Model file for the job. Use its own axes, mm. Coordinates: 2 decimals unless noted, no trailing zeros. Write each loop counter-clockwise with the first axis right and the second up, starting at its lowest first coordinate (ties: lowest second). Pieces come first, ordered by that corner, then holes.
Q1. Pull direction Y, two halves, no side cores. Call faces 1 (the flat face through (99, 0, 2)), 2 (the flat face through (99, 41, 2)), 3 (the flat face through (99, 41, 0)), 4 (the flat face through (99, 80, 2)): released by +Y, released by -Y, zero draft, split by the parting line, or undercut.
Q2. Drill centre lines: probe 1 along X at (y, z) = (64, 1.7); probe 2 along Y at (x, z) = (36, 3.35); probe 3 along Z at (x, y) = (10, 45). Where is each one in solid material? Low to high.
Q3. Band-saw the part on A-A, the plane y = 10. Write the cut outline in (x, z), plus the area to 3 significant figures.
Q4. Band-saw the part on B-B, the plane z = 2.65. Write the cut outline in (x, y).
Q5. Band-saw the part on C-C, the plane x = 116. State how many separate pieces and enclosed holes the cut face has, plus the area to 3 significant figures.
from build123d import *

# Parameters (mm, degrees)
SKETCH_W      = 200
SKETCH_H      = 80
PAD_DEPTH     = 2
SKETCH001_W   = 158
SKETCH001_H   = 2
SKETCH001_W_2 = 156.797272
PAD001_DEPTH  = 2
SKETCH002_W   = 166
SKETCH002_H   = 8
SKETCH002_H_2 = 10
SKETCH002_H_3 = 12
SKETCH002_W_2 = 20
SKETCH002_H_4 = 4
SKETCH002_W_3 = 16
SKETCH002_W_4 = 22
SKETCH002_W_5 = 14
SKETCH002_W_6 = 18
SKETCH002_W_7 = 12
SKETCH002_H_5 = 6
POCKET_DEPTH  = 5


with BuildPart() as part:
    # Sketch → Pad (new body)
    with BuildSketch(Plane.XY):
        with Locations((100, 40)):
            Rectangle(SKETCH_W, SKETCH_H)
    extrude(amount=PAD_DEPTH)

    # Sketch001 (on Face6 of Pad) → Pad001 (join)
    with BuildSketch(Plane.XY.offset(2)):
        with Locations((101, 1)):
            Rectangle(SKETCH001_W, SKETCH001_H)
        with Locations((100.398636, 79)):
            Rectangle(SKETCH001_W_2, SKETCH001_H)
    extrude(amount=PAD001_DEPTH)

    # Sketch002 (on Face5 of Pad001) → Pocket (cut)
    with BuildSketch(Plane.XY.offset(2)):
        with Locations((99, 72)):
            Rectangle(SKETCH002_W, SKETCH002_H)
        with Locations((99, 61)):
            Rectangle(SKETCH002_W, SKETCH002_H_2)
        with Locations((99, 48)):
            Rectangle(SKETCH002_W, SKETCH002_H_3)
        with Locations((99, 8)):
            Rectangle(SKETCH002_W, SKETCH002_H)
        with Locations((26, 16)):
            Rectangle(SKETCH002_W_2, SKETCH002_H_4)
        with Locations((48, 16)):
            Rectangle(SKETCH002_W_3, SKETCH002_H_4)
        with Locations((73, 16)):
            Rectangle(SKETCH002_W_4, SKETCH002_H_4)
        with Locations((95, 16)):
            Rectangle(SKETCH002_W_5, SKETCH002_H_4)
        with Locations((115, 16)):
            Rectangle(SKETCH002_W_6, SKETCH002_H_4)
        with Locations((137, 16)):
            Rectangle(SKETCH002_W_6, SKETCH002_H_4)
        with Locations((156, 16)):
            Rectangle(SKETCH002_W_7, SKETCH002_H_4)
        with Locations((174, 16)):
            Rectangle(SKETCH002_W_3, SKETCH002_H_4)
        with Locations((99, 25)):
            Rectangle(SKETCH002_W, SKETCH002_H_5)
        with Locations((99, 35)):
            Rectangle(SKETCH002_W, SKETCH002_H_5)
    extrude(amount=-POCKET_DEPTH, mode=Mode.SUBTRACT)


solid = part.part
Answer sheet:
1. face 1: released by -Y
1. face 2: undercut
1. face 3: zero draft
1. face 4: released by +Y
2. probe 1: x = 0 to 16, 182 to 200
2. probe 2: y = 0 to 2, 78 to 80
2. probe 3: z = 0 to 2
3. outline: (0, 0) - (16, 0) - (16, 2) - (0, 2) - close; (182, 0) - (200, 0) - (200, 2) - (182, 2) - close
3. area: 68.0 mm2
4. outline: (22, 0) - (180, 0) - (180, 2) - (22, 2) - close; (22, 78) - (178.8, 78) - (178.8, 80) - (22, 80) - close
5. separate pieces: 8
5. enclosed holes: 0
5. area: 60.0 mm2
